from build123d import *

# Parameters (mm, degrees)
SKETCH_1_R               = 10
SKETCH_1_R_2             = 2.5
EXTRUDE_1_DEPTH          = 70
SKETCH_2_W               = 60
SKETCH_2_H               = 70
SKETCH_2_H_2             = 67.94057246
CUT_EXTRUDE_1_DEPTH      = 70
EXTRUDE_2_DEPTH          = 60
CUT_EXTRUDE_3_DEPTH      = 129.790186287
CUT_EXTRUDE_3_DEPTH_BACK = 129.790186287
SKETCH_6_R               = 2.5
CUT_EXTRUDE_4_DEPTH      = 132.384596068
CUT_EXTRUDE_4_DEPTH_BACK = 132.384596068
SKETCH_7_W               = 40.15837314
SKETCH_7_H               = 126.534822783
SKETCH_7_W_2             = 29.990396309
SKETCH_7_H_2             = 127.151063803
SKETCH_8_R               = 2.5
EXTRUDE_4_DEPTH          = 2


with BuildPart() as part:
    # Sketch 1 → Extrude 1 (new body)
    with BuildSketch(Plane.XY):
        with BuildLine():
            Line((-15, 90), (-15, 0))
            ThreePointArc((-15, 0), (0, -15), (15, 0))
            Line((15, 0), (15, 90))
            ThreePointArc((15, 90), (0, 105), (-15, 90))
        make_face()
        Circle(SKETCH_1_R, mode=Mode.SUBTRACT)
        with Locations((0, 90)):
            Circle(SKETCH_1_R_2, mode=Mode.SUBTRACT)
    extrude(amount=EXTRUDE_1_DEPTH)

    # Sketch 2 → Cut-Extrude 1 (cut)
    with BuildSketch(Plane.ZY.offset(15)):
        with Locations((35, 80)):
            Rectangle(SKETCH_2_W, SKETCH_2_H)
        with Locations((35, 11.02971377)):
            Rectangle(SKETCH_2_W, SKETCH_2_H_2)
    extrude(amount=-CUT_EXTRUDE_1_DEPTH, mode=Mode.SUBTRACT)


with BuildPart() as cut_extrude_1_piece_1:
    # of the separate pieces the step leaves, piece 1, a body of its own (cut_extrude_1_pieces)
    add(part.part.solids().sort_by_distance((15, 0, 0))[0])



with BuildPart() as cut_extrude_1_piece_2:
    # of the separate pieces the step leaves, piece 2, a body of its own (cut_extrude_1_pieces)
    add(part.part.solids().sort_by_distance((15, 0, 65))[0])


with BuildPart() as cut_extrude_1_piece_1_1:
    add(cut_extrude_1_piece_1.part)

    add(cut_extrude_1_piece_2.part)  # Extrude 2 merges Cut-Extrude 1 piece 2
    # Sketch 4 → Extrude 2 (add)
    with BuildSketch(Plane(origin=(0, 0, 65), x_dir=(-1, 0, 0), z_dir=(0, 0, -1))):
        with BuildLine():
            Line((-4.490156776, 68.758657712), (15, 57.50601045))
            Line((15, 57.50601045), (36.319312502, 12.911360415))
            ThreePointArc((36.319312502, 12.911360415), (35.142094618, 9.577570071), (31.808304274, 10.754787955))
            Line((31.808304274, 10.754787955), (15, 45.913541163))
            Line((15, 45.913541163), (-9.509843224, 60.064305746))
            ThreePointArc((-9.509843224, 60.064305746), (-11.347175983, 66.921324953), (-4.490156776, 68.758657712))
        make_face()
    extrude(amount=EXTRUDE_2_DEPTH)

    # Sketch 6 → Cut-Extrude 3 (cut, two sides: drawn at the far end of the back side and taken through both)
    with BuildSketch(Plane(origin=(0, 0, 65), x_dir=(-1, 0, 0), z_dir=(0, 0, -1)).offset(-CUT_EXTRUDE_3_DEPTH_BACK)):
        with Locations(Location((-7, 64.411481729, 0), (0, 0, 90))):
            Circle(SKETCH_6_R)
        with Locations(Location((-11.650635095, 53.212249296, 0), (0, 0, 90))):
            Circle(SKETCH_6_R)
        with Locations(Location((10, 40.712249296, 0), (0, 0, 90))):
            Circle(SKETCH_6_R)
        with Locations(Location((10.320508076, 54.411481729, 0), (0, 0, 90))):
            Circle(SKETCH_6_R)
    extrude(amount=CUT_EXTRUDE_3_DEPTH + CUT_EXTRUDE_3_DEPTH_BACK, mode=Mode.SUBTRACT)

    # Sketch 7 → Cut-Extrude 4 (cut, two sides: drawn at the far end of the back side and taken through both)
    with BuildSketch(Plane(origin=(0, 0, 0), x_dir=(0, 0, -1), z_dir=(1, 0, 0)).offset(-CUT_EXTRUDE_4_DEPTH_BACK)):
        with Locations((15.07918657, 44.332405561)):
            Rectangle(SKETCH_7_W, SKETCH_7_H)
        with Locations((-79.995198155, 44.024285052)):
            Rectangle(SKETCH_7_W_2, SKETCH_7_H_2)
    extrude(amount=CUT_EXTRUDE_4_DEPTH + CUT_EXTRUDE_4_DEPTH_BACK, mode=Mode.SUBTRACT)

    # Sketch 8 → Extrude 4 (add)
    with BuildSketch(Plane(origin=(0, 0, 5), x_dir=(-1, 0, 0), z_dir=(0, 0, -1))):
        with BuildLine():
            Line((36.319312502, 12.911360415), (15, 57.50601045))
            Line((15, 57.50601045), (-4.490156776, 68.758657712))
            ThreePointArc((-4.490156776, 68.758657712), (-11.347175983, 66.921324953), (-9.509843224, 60.064305746))
            Line((-9.509843224, 60.064305746), (15, 45.913541163))
            Line((15, 45.913541163), (31.808304274, 10.754787955))
            ThreePointArc((31.808304274, 10.754787955), (35.142094618, 9.577570071), (36.319312502, 12.911360415))
        make_face()
        with Locations(Location((-7, 64.411481729, 0), (0, 0, 90))):
            Circle(SKETCH_8_R, mode=Mode.SUBTRACT)
        with Locations(Location((10.320508076, 54.411481729, 0), (0, 0, 90))):
            Circle(SKETCH_8_R, mode=Mode.SUBTRACT)
    extrude(amount=EXTRUDE_4_DEPTH)


solid = cut_extrude_1_piece_1_1.part
Build history of the part. All positions in model axes, mm. Coordinates: 2 decimals unless noted, no trailing zeros. Order: outer loops, then holes, each group sorted by start corner. A loop starts at its lowest first (then second) coordinate and runs counter-clockwise, first axis right, second up. Notation, with made-up numbers: M 5,68 L 56,68 A36 ccw 56,104 Z; hole C -2.5,5.5 d4. An arc over 180 degrees is marked long. One line per question, with ' | ' between items. Start each with the question number.
Q1. Saw through at A-A (x = 7). List the corners of the cut face in (y, z), then the cut area to 3 significant figures.
Q2. Saw through at C-C (x = -6). List the corners of the cut face in (y, z).
Q3. Saw through at D-D (y = 20.5). List the corners of the cut face in (x, z).
Q4. Two-plate mould, pull along Y, no slides. Class faces 1 (the face through (-11.28, 56.72, 34.43)), 2 (the face through (-23.286, 28.58, 34.434)), 3 (the face through (-16, 46, 65)): +Y half, -Y half, draft (parallel to the pull), parting line (faces both ways), or undercut.
Q5. Flat gauge pins, fed straight in: pin 1 Ø12 at (x, z) = (-8.5, 21.5) entering from +Y; pin 2 Ø5 at (y, z) = (35.5, 27.5) entering from -X; pin 3 Ø4 at (y, z) = (54, 50.5) entering from -X. Where does each tip first touch, or does it go through?
Q6. Saw through at B-B (z = 30). List the corners of the cut face in (x, y).
Q7. Probe L1, parallel to Y at x = 7, z = 31; L2, parallel to X at y = 52.5, z = 54.5; L3, parallel to X at y = 64.5, z = 37. List the from-to ranges inside material, lowest first. Write a range as from..to.
Check values:
1) outline: M 58.62,3 L 61.91,3 L 61.91,65 L 58.62,65 Z; M 66.91,3 L 69.43,3 L 69.43,65 L 66.91,65 Z | area: 361 mm2
2) outline: M 51.11,3 L 62.7,3 L 62.7,65 L 51.11,65 Z
3) outline: M -32.69,3 L -27.15,3 L -27.15,65 L -32.69,65 Z
4) face 1: undercut | face 2: -Y half | face 3: draft
5) pin 1: stops at y = 64.72 | pin 2: stops at x = -26.72 | pin 3: stops at x = -17.63
6) outline: M -36.32,12.91 A2.5 ccw -31.81,10.75 L -15,45.91 L 9.51,60.06 A5.02 ccw 4.49,68.76 L -15,57.51 Z; hole C -10.32,54.41 d5; hole C 7,64.41 d5
7) L1: y = 58.62..61.91, 66.91..69.43 | L2: x = -17.39..-11.93, -8.71..-3.59 | L3: x = -2.89..4.5, 9.5..12.02
